Geometry check sheet. Reference: the model listing, model coordinates, mm. Face numbers are marked on the shaded views. A direction names the side the tool comes from. Give positions to 0.01 mm unless a question says otherwise; leave off trailing zeros. Order: outer loops, then holes, each group sorted by start corner. A loop starts at its lowest first (then second) coordinate and runs counter-clockwise, first axis right, second up. Notation, with made-up numbers: M -5,70 L 7,70 A22 cw 7,107 Z; hole C 32,-13 d5. An arc over 180 degrees is marked long. Use CSV: the item, a comma, the result in double quotes. Start each with the question number.
from build123d import *

# Parameters (mm, degrees)
F0_W          = 203.2
F0_H          = 609.6
F1_DEPTH      = 12.7
F2_W          = 203.2
F2_H          = 18.7501087368
F3_DEPTH      = 660.4
F5_DEPTH      = 10.16
F5_DEPTH_BACK = 579.12


with BuildPart() as f1:
    # F0 (on Top) → F1 (new body)
    with BuildSketch(Plane.XY):
        with Locations((-26.7803451535, 0.5164034665)):
            Rectangle(F0_W, F0_H)
    extrude(amount=F1_DEPTH)

    # F2 (on face) → F3 (join)
    with BuildSketch(Plane.XY.offset(12.7)):
        with Locations((-26.7803451535, 294.9085421652)):
            Rectangle(F2_W, F2_H)
        with Locations((-26.7803451535, -294.9085421652)):
            Rectangle(F2_W, F2_H)
    extrude(amount=F3_DEPTH)

    # F4 (on face) → F5 (cut, two sides)
    with BuildSketch(Plane(origin=(0, -285.5334877968, 0), x_dir=(-1, 0, 0), z_dir=(0, 1, 0))) as f5_sk:
        with BuildLine():
            Line((-47.3919240568, 558.3197568053), (-47.3919240568, 127.4802431947))
            ThreePointArc((-47.3919240568, 127.4802431947), (-47.3919755667, 127.3792859835), (-47.3918984296, 127.2783287887))
            ThreePointArc((-47.3918984296, 127.2783287887), (31.835410726, 48.161954644), (111.0627199175, 127.2783287527))
            ThreePointArc((111.0627199175, 127.2783287527), (111.0627976927, 127.3893415928), (111.0627199175, 127.5003544328))
            Line((111.0627199175, 127.5003544328), (111.0627199175, 558.2996455672))
            ThreePointArc((111.0627199175, 558.2996455672), (111.0627970546, 558.4006027949), (111.0627455447, 558.5015600389))
            ThreePointArc((111.0627455447, 558.5015600389), (31.835410729, 637.638045356), (-47.3919240568, 558.5015600091))
            ThreePointArc((-47.3919240568, 558.5015600091), (-47.3919762048, 558.4106584072), (-47.3919240568, 558.3197568053))
        make_face()
        with BuildLine():
            ThreePointArc((-36.7020475123, 127.2783288007), (-36.7021366804, 127.3792859868), (-36.7020771365, 127.4802431948))
            Line((-36.7020771365, 127.4802431948), (-36.7020771365, 558.3197568053))
            ThreePointArc((-36.7020771365, 558.3197568053), (-36.7021374181, 558.4106584072), (-36.7020771365, 558.5015600091))
            ThreePointArc((-36.7020771365, 558.5015600091), (31.8354107241, 626.9482065693), (100.3728986244, 558.5015600488))
            ThreePointArc((100.3728986244, 558.5015600488), (100.3729581683, 558.400602797), (100.3728690001, 558.2996455671))
            Line((100.3728690001, 558.2996455671), (100.3728690001, 127.5003544328))
            ThreePointArc((100.3728690001, 127.5003544328), (100.372958906, 127.3893415928), (100.3728690001, 127.2783287527))
            ThreePointArc((100.3728690001, 127.2783287527), (31.83541072, 58.8517934307), (-36.7020475123, 127.2783288007))
        make_face(mode=Mode.SUBTRACT)
    extrude(amount=-F5_DEPTH, mode=Mode.SUBTRACT)
    extrude(f5_sk.sketch, amount=F5_DEPTH_BACK, mode=Mode.SUBTRACT)


solid = f1.part
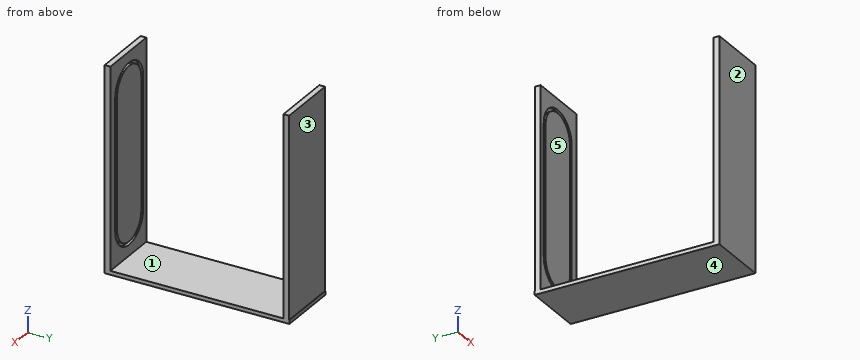
(1) Sectioned sample at D-D on y = -10.5. Record the cut outline in (x, z), then the cut area to 3 significant figures.
(2) Sectioned sample at A-A on z = 255.5. Record the cut outline in (x, y), then the cut area to 3 significant figures.
(3) Access from +Z, -Z, +X, -X, +Y, -Y to the whole of each face (thin tool, end or side, straight path). Record for the marked faces 1 and 2.
(4) Thickness scan on line 1 (Y direction, x = -32, z = 121); line 2 (Z direction, x = -114.5, y = 39.5); line 3 (Y direction, x = -3.5, z = 62). Record the ranges inside material, lowest first.
(5) Sectioned sample at C-C on z = 118. Record the cut outline in (x, y), then the cut area to 3 significant figures.
(6) Go/stop test with flat-tipped pins: P1, Ø1, axis at x = 46, y = -182.5, coming from the +Z side; P2, Ø1, axis at x = -80.5, z = 127.5, coming from the +Y side. Record where each tip stops, or that it passes through.
(7) Draft check along Y on the marked faces 3, 4 and 5. Enter one of: +Y half, -Y half, draft (parallel to the pull), parting line (faces both ways), or undercut.
(8) Sectioned sample at B-B on x = -89. Record the cut outline in (y, z), then the cut area to 3 significant figures.
Responses:
1,outline,"M -128.38,0 L 74.82,0 L 74.82,12.7 L -128.38,12.7 Z"
1,area,"2,580 mm2"
2,outline,"M -128.38,-304.28 L 74.82,-304.28 L 74.82,-285.53 L 47.39,-285.53 L 47.39,-295.69 L 36.7,-295.69 L 36.7,-285.53 L -100.37,-285.53 L -100.37,-295.69 L -111.06,-295.69 L -111.06,-285.53 L -128.38,-285.53 Z; M -128.38,285.53 L -111.06,285.53 L -111.06,293.59 L -100.37,293.59 L -100.37,285.53 L 36.7,285.53 L 36.7,293.59 L 47.39,293.59 L 47.39,285.53 L 74.82,285.53 L 74.82,304.28 L -128.38,304.28 Z"
2,area,"7,230 mm2"
3,face 1,"+Z, +X, -X"
3,face 2,"+Z, -Z, +X, -X, -Y"
4,line 1,"-304.28 to -285.53, 285.53 to 304.28"
4,line 2,"0 to 12.7"
4,line 3,"-304.28 to -295.69, 293.59 to 304.28"
5,outline,"M -128.38,-304.28 L 74.82,-304.28 L 74.82,-285.53 L 46.83,-285.53 L 46.83,-295.69 L 36.06,-295.69 L 36.06,-285.53 L -99.73,-285.53 L -99.73,-295.69 L -110.5,-295.69 L -110.5,-285.53 L -128.38,-285.53 Z; M -128.38,285.53 L -110.5,285.53 L -110.5,293.59 L -99.73,293.59 L -99.73,285.53 L 36.06,285.53 L 36.06,293.59 L 46.83,293.59 L 46.83,285.53 L 74.82,285.53 L 74.82,304.28 L -128.38,304.28 Z"
5,area,"7,230 mm2"
6,P1,"z = 12.7"
6,P2,"y = 304.28"
7,face 3,"+Y half"
7,face 4,"draft"
7,face 5,"undercut"
8,outline,"M -304.28,0 L 305.32,0 L 305.32,12.7 L 304.28,12.7 L 304.28,673.1 L 285.53,673.1 L 285.53,613.27 L 293.59,613.27 L 293.59,596.22 L 285.53,596.22 L 285.53,89.58 L 293.59,89.58 L 293.59,72.53 L 285.53,72.53 L 285.53,12.7 L -285.53,12.7 L -285.53,72.53 L -295.69,72.53 L -295.69,89.58 L -285.53,89.58 L -285.53,596.22 L -295.69,596.22 L -295.69,613.27 L -285.53,613.27 L -285.53,673.1 L -304.28,673.1 Z"
8,area,"31,900 mm2"
